from build123d import *

# Parameters (mm, degrees)
F1_DEPTH = 285.75
F2_W     = 11.1125
F2_H     = 11.1125
F2_R     = 3.175
F3_DEPTH = 50.801


with BuildPart() as f1:
    # F0 (on Top) → F1 (new body, symmetric)
    with BuildSketch(Plane.XY):
        Polygon((-2.54, 50.8), (-2.54, 2.54), (-76.2, 2.54), (-76.2, 0), (0, 0), (0, 48.26), (35.56, 48.26), (35.56, 50.8), align=None)
    extrude(amount=F1_DEPTH, both=True)

    # F2 (on face) → F3 (cut, through all)
    with BuildSketch(Plane.XZ):
        with Locations((-50.8, 266.7)):
            Rectangle(F2_W, F2_H)
        with Locations((-50.8, -266.7)):
            Rectangle(F2_W, F2_H)
        with Locations((19.05, 254)):
            Circle(F2_R)
        with Locations((19.05, 0)):
            Circle(F2_R)
        with Locations((19.05, -254)):
            Circle(F2_R)
    extrude(amount=-F3_DEPTH, mode=Mode.SUBTRACT)


solid = f1.part
Design review of the part built by this model. Coordinates are the model's own, in mm. A direction names the side the tool comes from. Round coordinates to 2 decimals unless told otherwise and drop trailing zeros. Write each loop counter-clockwise with the first axis right and the second up, starting at its lowest first coordinate (ties: lowest second). Pieces come first, ordered by that corner, then holes. Notation, with made-up numbers: (67, 42.5) - (114, 42.5) arc R13 cw to (114, 47.5) - close; hole circle Ø6 at (63, 12). An arc over 180 degrees is marked (long way). Return JSON: item names as keys, results as strings. Group by question number.
Item 1: We need section C-C on y = 17. Write out the cut boundary in (x, z).
Item 2: We need section B-B on x = -26. Write out the cut boundary in (y, z), and give its area (3 significant figures).
Item 3: For probe 1 along Z at (x, y) = (19.05, 50) (3 decimals); probe 2 along X at (y, z) = (49.2, -254) (3 decimals); probe 3 along X at (y, z) = (45.5, -71.5), list the stretches that pass through material, from the lowest coordinate up. Write a range as [from, to].
Item 4: Insertion check: P1, Ø24, axis at y = 26, z = 106, coming from the +X side; P2, Ø5.5, axis at x = 19.05, z = 254, coming from the +Y side; P3, Ø1.5, axis at y = 5.5, z = 107, coming from the -X side; P4, Ø22, axis at x = -34, z = 6.5, coming from the +Y side. Each pin has a flat end and moves straight along its axis. Give the tip position at first contact, or say it passes through.
Item 5: We need section A-A on z = 242.5. Write out the cut boundary in (x, y).
Item 6: Machinability: for faces 1 (the face through (17, 50.8, 4)), 2 (the face through (18, 48.26, 4)), 3 (the face through (-2.54, 27, 4)), which of the approach directions +Z, -Z, +X, -X, +Y, -Y give a long, thin tool a straight path to every point of the face, cutting with its end or side? Answer none if there is none.
Model answer:
{
 "1": {"outline": "(-2.54, -285.75) - (0, -285.75) - (0, 285.75) - (-2.54, 285.75) - close"},
 "2": {"outline": "(0, -285.75) - (2.54, -285.75) - (2.54, 285.75) - (0, 285.75) - close", "area": "1,450 mm²"},
 "3": {"probe 1": "z = [-285.75, -257.175], [-250.825, -3.175], [3.175, 250.825], [257.175, 285.75]", "probe 2": "x = [-2.54, 15.875], [22.225, 35.56]", "probe 3": "x = [-2.54, 0]"},
 "4": {"P1": "stops at x = 0", "P2": "passes through", "P3": "stops at x = -2.54", "P4": "stops at y = 2.54"},
 "5": {"outline": "(-76.2, 0) - (0, 0) - (0, 48.26) - (35.56, 48.26) - (35.56, 50.8) - (-2.54, 50.8) - (-2.54, 2.54) - (-76.2, 2.54) - close"},
 "6": {"face 1": "+Z, -Z, +X, -X, +Y", "face 2": "+Z, -Z, +X, -Y", "face 3": "+Z, -Z, -X, +Y"}
}
